Verification items for the finished model (mm, model axes). A direction names the side the tool comes from. Round coordinates to 2 decimals unless told otherwise and drop trailing zeros. Write each loop counter-clockwise with the first axis right and the second up, starting at its lowest first coordinate (ties: lowest second). Pieces come first, ordered by that corner, then holes. Notation, with made-up numbers: M 39,41 L 86,41 A7 ccw 86,46 Z; hole C 64.5,-5.75 d10. An arc over 180 degrees is marked long. One line per question, with ' | ' between items.
from build123d import *

# Parameters (mm, degrees)
SKETCH1_W           = 304.8
SKETCH1_H           = 101.6
BOSS_EXTRUDE1_DEPTH = 6.35
SKETCH2_R           = 12.7
BOSS_EXTRUDE3_DEPTH = 5.55625
SKETCH9_R           = 11.1125
CUT_EXTRUDE4_DEPTH  = 4.445
CUT_EXTRUDE5_START  = -5.55625
SKETCH10_R          = 11.1125
CUT_EXTRUDE5_DEPTH  = 5.55625
SKETCH11_R          = 7.9375
CUT_EXTRUDE6_DEPTH  = 310.094403462
SKETCH12_R          = 12.7
CUT_EXTRUDE7_DEPTH  = 310.0695755
SKETCH22_W          = 63.5
SKETCH22_H          = 63.5
BOSS_EXTRUDE7_DEPTH = 12.7
SKETCH25_W          = 50.8
SKETCH25_H          = 50.8
CUT_EXTRUDE11_DEPTH = 15.875
SKETCH18_W          = 40.386
SKETCH18_H          = 20.066
BOSS_EXTRUDE5_DEPTH = 39.878
SKETCH32_R          = 4.7625
CUT_EXTRUDE12_DEPTH = 6.35
SKETCH34_W          = 36.133088602
SKETCH34_H          = 18.470251096
CUT_EXTRUDE13_DEPTH = 312.566902742


with BuildPart() as part:
    # Sketch1 → Boss-Extrude1 (new body)
    with BuildSketch(Plane(origin=(0, 0, 0), x_dir=(1, 0, 0), z_dir=(0, 1, 0))):
        with Locations((-152.4, 0)):
            Rectangle(SKETCH1_W, SKETCH1_H)
    extrude(amount=BOSS_EXTRUDE1_DEPTH)

    # Sketch2 → Boss-Extrude3 (add)
    with BuildSketch(Plane(origin=(0, 6.35, 0), x_dir=(1, 0, 0), z_dir=(0, 1, 0))):
        with Locations(Location((-258.510557857, 0, 0), (0, 0, 90))):
            Circle(SKETCH2_R)
    extrude(amount=BOSS_EXTRUDE3_DEPTH)

    # Sketch9 → Cut-Extrude4 (cut)
    with BuildSketch(Plane(origin=(0, 11.90625, 0), x_dir=(1, 0, 0), z_dir=(0, 1, 0))):
        with Locations(Location((-258.510557857, 0, 0), (0, 0, 270))):
            Circle(SKETCH9_R)
    extrude(amount=-CUT_EXTRUDE4_DEPTH, mode=Mode.SUBTRACT)

    # Sketch10 → Cut-Extrude5 (cut)
    with BuildSketch(Plane(origin=(0, 0, 0), x_dir=(-1, 0, 0), z_dir=(0, -1, 0)).offset(CUT_EXTRUDE5_START)):
        with Locations(Location((258.510557857, 0, 0), (0, 0, 270))):
            Circle(SKETCH10_R)
    extrude(amount=CUT_EXTRUDE5_DEPTH, mode=Mode.SUBTRACT)

    # Sketch11 → Cut-Extrude6 (cut, through all)
    with BuildSketch(Plane(origin=(0, 7.46125, 0), x_dir=(1, 0, 0), z_dir=(0, 1, 0))):
        with Locations(Location((-258.510557857, 0, 0), (0, 0, 270))):
            Circle(SKETCH11_R)
    extrude(amount=-CUT_EXTRUDE6_DEPTH, mode=Mode.SUBTRACT)

    # Sketch12 → Cut-Extrude7 (cut, through all)
    with BuildSketch(Plane(origin=(0, 6.35, 0), x_dir=(1, 0, 0), z_dir=(0, 1, 0))):
        with Locations(Location((-134.666203771, 0, 0), (0, 0, 270))):
            Circle(SKETCH12_R)
    extrude(amount=-CUT_EXTRUDE7_DEPTH, mode=Mode.SUBTRACT)

    # Sketch22 → Boss-Extrude7 (add)
    with BuildSketch(Plane(origin=(0, 6.35, 0), x_dir=(1, 0, 0), z_dir=(0, 1, 0))):
        with Locations((-134.666203771, 0)):
            Rectangle(SKETCH22_W, SKETCH22_H)
    extrude(amount=BOSS_EXTRUDE7_DEPTH)

    # Sketch25 → Cut-Extrude11 (cut)
    with BuildSketch(Plane(origin=(0, 19.05, 0), x_dir=(1, 0, 0), z_dir=(0, 1, 0))):
        with Locations((-134.666203771, 0)):
            Rectangle(SKETCH25_W, SKETCH25_H)
    extrude(amount=-CUT_EXTRUDE11_DEPTH, mode=Mode.SUBTRACT)

    # Sketch18 → Boss-Extrude5 (add)
    with BuildSketch(Plane(origin=(0, 6.35, 0), x_dir=(1, 0, 0), z_dir=(0, 1, 0))):
        with Locations((-206.419013169, 0)):
            Rectangle(SKETCH18_W, SKETCH18_H)
    extrude(amount=BOSS_EXTRUDE5_DEPTH)

    # Sketch32 → Cut-Extrude12 (cut)
    with BuildSketch(Plane(origin=(0, 6.35, 0), x_dir=(1, 0, 0), z_dir=(0, 1, 0))):
        with Locations(Location((-7.62, -42.893773539, 0), (0, 0, 270))):
            Circle(SKETCH32_R)
        with Locations(Location((-21.59, -42.893773539, 0), (0, 0, 270))):
            Circle(SKETCH32_R)
        with Locations(Location((-7.62, 42.272941973, 0), (0, 0, 270))):
            Circle(SKETCH32_R)
        with Locations(Location((-21.59, 42.272941973, 0), (0, 0, 270))):
            Circle(SKETCH32_R)
    extrude(amount=-CUT_EXTRUDE12_DEPTH, mode=Mode.SUBTRACT)

    # Sketch34 → Cut-Extrude13 (cut, through all)
    with BuildSketch(Plane(origin=(0, 6.35, 0), x_dir=(1, 0, 0), z_dir=(0, 1, 0))):
        with Locations((-18.066544301, -24.7777)):
            Rectangle(SKETCH34_W, SKETCH34_H)
    extrude(amount=-CUT_EXTRUDE13_DEPTH, mode=Mode.SUBTRACT)


solid = part.part
1. Section check D-D, the plane z = -21.5. Record the cut outline in (x, y) (3 decimals).
Results:
outline: M -304.8,0 L 0,0 L 0,6.35 L -102.916,6.35 L -102.916,19.05 L -109.266,19.05 L -109.266,3.175 L -160.066,3.175 L -160.066,19.05 L -166.416,19.05 L -166.416,6.35 L -304.8,6.35 Z
2. Thickness scan on line 1 (X direction, y = 10.3, z = 0); line 2 (X direction, y = 1.95, z = 0); line 3 (X direction, y = 7.5, z = -9). Record the ranges inside material, lowest first.
Results:
line 1: x = -271.21 to -269.62, -247.4 to -245.81, -226.61 to -186.23, -166.42 to -160.07, -109.27 to -102.92 | line 2: x = -304.8 to -269.62, -247.4 to -147.37, -121.97 to 0 | line 3: x = -267.47 to -265.03, -251.99 to -249.55, -226.61 to -186.23, -166.42 to -160.07, -109.27 to -102.92
3. Section check C-C, the plane x = -254.5. Record the cut outline in (y, z).
Results:
outline: M 0,-50.8 L 6.35,-50.8 L 6.35,-12.05 L 11.91,-12.05 L 11.91,-10.36 L 7.46,-10.36 L 7.46,-6.85 L 5.56,-6.85 L 5.56,-10.36 L 0,-10.36 Z; M 0,10.36 L 5.56,10.36 L 5.56,6.85 L 7.46,6.85 L 7.46,10.36 L 11.91,10.36 L 11.91,12.05 L 6.35,12.05 L 6.35,50.8 L 0,50.8 Z
4. Mould release check, pull along Z, two halves, no side actions. Record for faces 4 (the face through (-247, 11.906, 0)), 5 (the face through (-256, 7.461, -8)): pulls with the +Z half, pulls with the -Z half, needs draft (parallel to the pull), parting line crosses it, or undercut.
Results:
face 4: needs draft | face 5: undercut
5. Tool access check on faces 1 (the face through (-18, 3, 34.013)), 2 (the face through (-186.226, 26, 0)), 3 (the face through (-269.36, 9.71, -2.41)). Record the directions out of +Z, -Z, +X, -X, +Y, -Y that give a thin tool (end or side, any length) a straight path to the whole face; none if there is none.
Results:
face 1: +X, +Y, -Y | face 2: +Z, -Z, +Y | face 3: +Y
6. Section check A-A, the plane x = -7.62. Record the cut outline in (y, z), then the cut area to 3 significant figures.
Results:
outline: M 0,-50.8 L 6.35,-50.8 L 6.35,-47.04 L 0,-47.04 Z; M 0,-37.51 L 6.35,-37.51 L 6.35,15.54 L 0,15.54 Z; M 0,34.01 L 6.35,34.01 L 6.35,38.13 L 0,38.13 Z; M 0,47.66 L 6.35,47.66 L 6.35,50.8 L 0,50.8 Z | area: 407 mm2
7. Section check B-B, the plane z = 41. Record the cut outline in (x, y).
Results:
outline: M -304.8,0 L -25.96,0 L -25.96,6.35 L -304.8,6.35 Z; M -17.22,0 L -11.99,0 L -11.99,6.35 L -17.22,6.35 Z; M -3.25,0 L 0,0 L 0,6.35 L -3.25,6.35 Z
8. Go/stop test with flat-tipped pins: P1, Ø6, axis at y = 30.5, z = -3.5, coming from the +X side; P2, Ø13.5, axis at x = -258.51, z = 0, coming from the +Y side; P3, Ø5, axis at y = 13, z = 8, coming from the -X side; P4, Ø8, axis at y = 17, z = 11, coming from the +X side. Record where each tip stops, or that it passes through.
Results:
P1: stops at x = -186.23 | P2: passes through | P3: stops at x = -269.83 | P4: stops at x = -102.92
